Design review of the part built by this model. Coordinates are the model's own, in mm. Round coordinates to 2 decimals unless told otherwise and drop trailing zeros. Order: outer loops, then holes, each group sorted by start corner. A loop starts at its lowest first (then second) coordinate and runs counter-clockwise, first axis right, second up. Notation, with made-up numbers: (83, 85.25) - (106, 85.25) arc R20 ccw to (106, 101.25) - close; hole circle Ø7 at (46.5, -26). An arc over 180 degrees is marked (long way). Use CSV: the item, a comma, the result in double quotes. Start each with the question number.
from build123d import *

# Parameters (mm, degrees)
BOSS_EXTRUDE1_DEPTH = 3.175


with BuildPart() as part:
    # Sketch1 → Boss-Extrude1 (new body)
    with BuildSketch(Plane.XY):
        Polygon((0, 0), (80, 0), (80, 65), (36.825, 65), (36.825, 61.825), (-36.825, 61.825), (-36.825, 65), (-80, 65), (-80, 0), align=None)
    extrude(amount=BOSS_EXTRUDE1_DEPTH)


solid = part.part
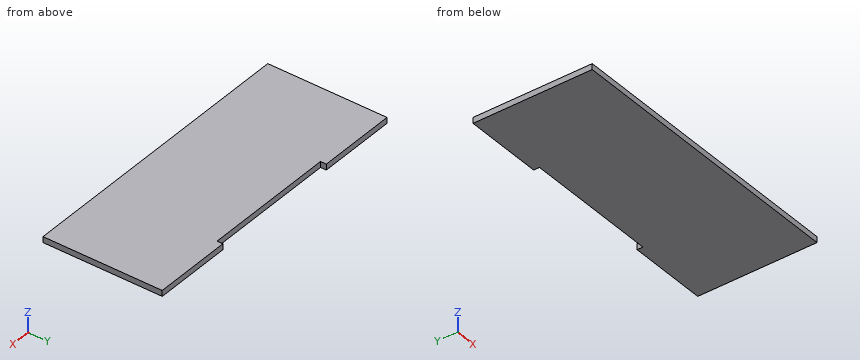
Q1. For L1, parallel to Y at x = 11.5, z = 1.95 (3 decimals), list the stretches that pass through material, from the lowest coordinate up. Write a range as [from, to].
Q2. Clearance check with a flat-ended pin moving along its axis: pin 1 (1 mm diameter, centred on x = -4.5, z = 1, fed in from +Y) (3 decimals). State where the tip first meets the part, or that it passes through.
Q3. Take a section at A-A (z = 0.85). State the section outline as (x, y) points (3 decimals), plus the area to 3 significant figures.
Q4. Take a section at B-B (x = -28). State the section outline as (y, z) points (3 decimals).
Findings below:
1,L1,"y = [0, 61.825]"
2,pin 1,"stops at y = 61.825"
3,outline,"(-80, 0) - (80, 0) - (80, 65) - (36.825, 65) - (36.825, 61.825) - (-36.825, 61.825) - (-36.825, 65) - (-80, 65) - close"
3,area,"10,200 mm^2"
4,outline,"(0, 0) - (61.825, 0) - (61.825, 3.175) - (0, 3.175) - close"
